For this review, take the finished solid that the model builds, in its own axes (mm). Face numbers are marked on the shaded views. Round coordinates to 2 decimals unless told otherwise and drop trailing zeros. Order: outer loops, then holes, each group sorted by start corner. A loop starts at its lowest first (then second) coordinate and runs counter-clockwise, first axis right, second up. Notation, with made-up numbers: (-13.75, -26) - (1.25, -26) arc R27 ccw to (1.25, 0) - close; hole circle Ø6 at (40, 15.25). An arc over 180 degrees is marked (long way). One line per item, written item: value.
```python
from build123d import *

# Parameters (mm, degrees)
F2_R      = 3.813781
F3_DEPTH  = 38.1
F4_R      = 3.020529
F5_DEPTH  = 14.0716
F3_FACE_R = 3.813781
F6_DEPTH  = 15.24


with BuildPart() as f1:
    # F0 (on Front) → F1 (revolve)
    with BuildSketch(Plane.XZ):
        Polygon((-1.911807, -2.718227), (1.97439, -2.723357), (1.97439, 2.356643), (22.062188, 17.901429), (18.175991, 22.923379), (-1.911807, 7.378592), align=None)
    revolve(axis=Axis((-1.911807, 0, 2.330183), (0, 0, -1)))

    # F2 (on Top) → F3 (cut)
    with BuildSketch(Plane.XY):
        with Locations((-1.898092, 0)):
            Circle(F2_R)
    extrude(amount=F3_DEPTH, mode=Mode.SUBTRACT)

    # F4 (on Top) → F5 (cut)
    with BuildSketch(Plane.XY):
        with Locations((-1.891657, 0)):
            Circle(F4_R)
    extrude(amount=F5_DEPTH, mode=Mode.SUBTRACT)

    # F3_face (on face) → F6 (cut)
    with BuildSketch(Plane(origin=(-1.898092, 0, 0), x_dir=(1, 0, 0), z_dir=(0, 0, 1))):
        Circle(F3_FACE_R)
    extrude(amount=-F6_DEPTH, mode=Mode.SUBTRACT)


solid = f1.part
```
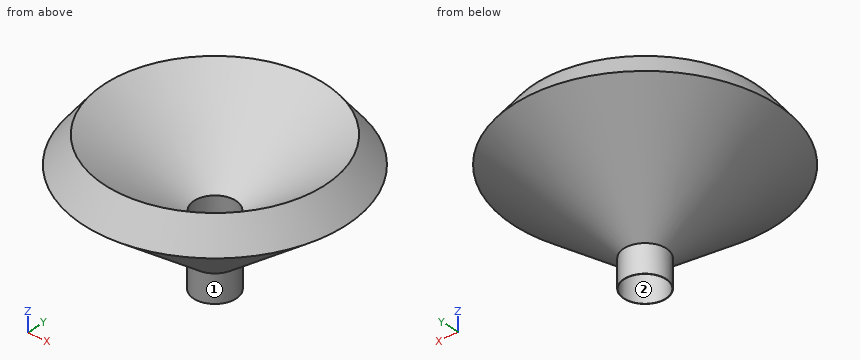
Item 1: For P1, Ø4, axis at x = 12.5, z = 15.5, coming from the -Y side; P2, Ø4, axis at x = -4, z = 0.5, coming from the +Y side; P3, Ø10, axis at x = 8, z = 8, coming from the +Y side, all flat-tipped, find the tip position at first contact; note any pin that passes through.
Returned:
P1: y = -18.84
P2: y = 3.89
P3: y = 15.18
Item 2: Take a section at B-B (z = 9.25). Write out the cut boundary in (x, y).
Returned:
outline: circle Ø25.59 at (-1.91, 0); hole circle Ø7.63 at (-1.9, 0)
Item 3: Wall thickness on line 1 (Y direction, x = -8, z = 17.5); line 2 (X direction, y = 0, z = 4.25); line 3 (X direction, y = 0, z = 2.75): over which ranges is each line inside the solid? List them lowest first.
Returned:
line 1: -22.65 to -11.58, 11.58 to 22.65
line 2: -8.24 to -5.71, 1.92 to 4.42
line 3: -6.31 to -5.71, 1.92 to 2.48
Item 4: The part is to be moulded in two halves that separate along X. For the marked faces 1 and 2, say which applies: +X half, -X half, draft (parallel to the pull), parting line (faces both ways), or undercut.
Returned:
face 1: parting line
face 2: undercut
Item 5: Take a section at A-A (y = 0). Write out the cut boundary in (x, z), plus the area to 3 significant figures.
Returned:
outline: (-25.89, 17.9) - (-5.8, 2.36) - (-5.8, -2.72) - (-5.71, -2.72) - (-5.71, 10.32) - (-22, 22.92) - close; (1.92, -2.72) - (1.97, -2.72) - (1.97, 2.36) - (22.06, 17.9) - (18.18, 22.92) - (1.92, 10.34) - close
area: 293 mm^2
